For this review, take the finished solid that the model builds, in its own axes (mm). Face numbers are marked on the shaded views. A direction names the side the tool comes from. Round coordinates to 2 decimals unless told otherwise and drop trailing zeros. Loops run counter-clockwise (first coordinate to the right, second up) from the corner with the lowest first, then second, coordinate; pieces in that order, holes last. Notation, with made-up numbers: (44, 48.25) -> (55, 48.25) arc R19 ccw to (55, 70.25) -> close; hole circle Ø8 at (28.25, 24). An arc over 180 degrees is marked (long way). One line per question, with ' | ' between items. Start each with the question number.
1. For pin 1 Ø4 at (x, y) = (-104, -81) entering from +Z; pin 2 Ø1.3 at (x, y) = (13.5, -102.5) entering from +Z; pin 3 Ø2 at (x, y) = (-11, 1) entering from +Z, all flat-tipped, find the tip position at first contact; note any pin that passes through.
2. Consider section A-A (z = 354.5). Write out the cut boundary in (x, y).
3. Consider section B-B (x = 35). Write out the cut boundary in (y, z), and give its area (3 significant figures).
4. Consider section C-C (y = -40). Write out the cut boundary in (x, z).
5. For the marked faces 4 and 5, list the 3-axis set-ups (+Z, -Z, +X, -X, +Y, -Y) from which the entire face can be reached by the end or side of a thin tool; tool diameter is ignored.
6. Draft analysis for pull direction X (two halves, no side actions). For the marked faces 1, 2 and 3, state which applies: pulls with the +X half, pulls with the -X half, needs draft (parallel to the pull), parting line crosses it, or undercut.
7. Wall thickness on line 1 along Y through (x, z) = (128.5, 18.5); line 2 along X through (y, z) = (-79, 129); line 3 along Y through (x, z) = (103, 344.5): over which ranges is each line inside the solid? List them lowest first.
8. Consider section D-D (z = 36). Write out the cut boundary in (x, y).
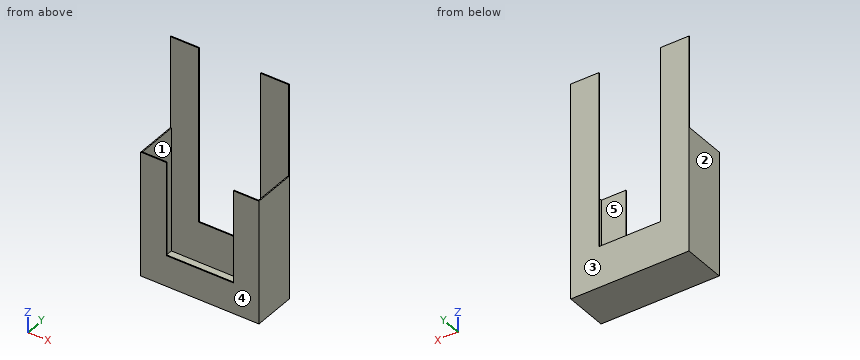
```python
from build123d import *

# Parameters (mm, degrees)
F0_W      = 292.1
F0_H      = 279.4
F1_DEPTH  = 2.54
F4_DEPTH  = 101.6
F5_W      = 63.5
F5_H      = 231.14
F5_H_2    = 76.2
F5_W_2    = 165.1
F5_H_3    = 228.6
F6_DEPTH  = 2.54
F7_W      = 292.1
F7_H      = 2.54
F8_DEPTH  = 25.4
F9_W      = 152.4
F9_H      = 431.8
F10_DEPTH = 25.4


with BuildPart() as f1:
    # F0 (on Front) → F1 (new body)
    with BuildSketch(Plane.XZ):
        Rectangle(F0_W, F0_H)
    extrude(amount=-F1_DEPTH)

    # F2: F1 across face


with BuildPart() as f1_1:
    add(f1.part)
    add(f1.part.mirror(Plane(origin=(0, 1.27, 139.7), x_dir=(1, 0, 0), z_dir=(0, 0, 1))))

    # F3 (on face) → F4 (join)
    with BuildSketch(Plane.XZ):
        Polygon((-143.51, -137.16), (-143.51, 167.64), (-146.05, 167.64), (-146.05, -139.7), (146.05, -139.7), (146.05, 165.1), (143.51, 165.1), (143.51, -137.16), align=None)
    extrude(amount=F4_DEPTH)

    # F5 (on face) → F6 (join)
    with BuildSketch(Plane.XZ.offset(101.6)):
        with Locations((-114.3, 52.07)):
            Rectangle(F5_W, F5_H)
        with Locations((-114.3, -101.6)):
            Rectangle(F5_W, F5_H_2)
        with Locations((0, -101.6)):
            Rectangle(F5_W_2, F5_H_2)
        with Locations((114.3, 50.8)):
            Rectangle(F5_W, F5_H_3)
        with Locations((114.3, -101.6)):
            Rectangle(F5_W, F5_H_2)
    extrude(amount=F6_DEPTH)

    # F7 (on face) → F8 (cut)
    with BuildSketch(Plane.XY.offset(419.1)):
        with Locations((0, 1.27)):
            Rectangle(F7_W, F7_H)
    extrude(amount=-F8_DEPTH, mode=Mode.SUBTRACT)

    # F9 (on face) → F10 (cut)
    with BuildSketch(Plane.XZ):
        with Locations((0, 177.8)):
            Rectangle(F9_W, F9_H)
    extrude(amount=-F10_DEPTH, mode=Mode.SUBTRACT)


solid = f1_1.part
```
Answer block:
1) pin 1: stops at z = -137.16 | pin 2: stops at z = -63.5 | pin 3: stops at z = -38.1
2) outline: (-146.05, 0) -> (-76.2, 0) -> (-76.2, 2.54) -> (-146.05, 2.54) -> close; (76.2, 0) -> (146.05, 0) -> (146.05, 2.54) -> (76.2, 2.54) -> close
3) outline: (-104.14, -139.7) -> (2.54, -139.7) -> (2.54, -38.1) -> (0, -38.1) -> (0, -137.16) -> (-101.6, -137.16) -> (-101.6, -63.5) -> (-104.14, -63.5) -> close | area: 710 mm2
4) outline: (-146.05, -139.7) -> (146.05, -139.7) -> (146.05, 165.1) -> (143.51, 165.1) -> (143.51, -137.16) -> (-143.51, -137.16) -> (-143.51, 167.64) -> (-146.05, 167.64) -> close
5) face 4: +Z, -Z, +X, -X, -Y | face 5: +Z
6) face 1: undercut | face 2: pulls with the -X half | face 3: needs draft
7) line 1: y = -104.14 to -101.6, 0 to 2.54 | line 2: x = -146.05 to -143.51, 143.51 to 146.05 | line 3: y = 0 to 2.54
8) outline: (-146.05, -104.14) -> (-82.55, -104.14) -> (-82.55, -101.6) -> (-143.51, -101.6) -> (-143.51, 0) -> (-76.2, 0) -> (-76.2, 2.54) -> (-146.05, 2.54) -> close; (76.2, 0) -> (143.51, 0) -> (143.51, -101.6) -> (82.55, -101.6) -> (82.55, -104.14) -> (146.05, -104.14) -> (146.05, 2.54) -> (76.2, 2.54) -> close
